```python
from build123d import *

# Parameters (mm, degrees)
F0_W     = 50.8
F0_H     = 38.1
F1_DEPTH = 25.4
F2_R     = 6.35
F3_DEPTH = 11.938
F4_R     = 8.89
F5_DEPTH = 6.35


with BuildPart() as f1:
    # F0 (on Front) → F1 (new body)
    with BuildSketch(Plane.XZ):
        with Locations((-25.4, -19.05)):
            Rectangle(F0_W, F0_H)
    extrude(amount=F1_DEPTH)

    # F2 (on Top) → F3 (join)
    with BuildSketch(Plane.XY):
        with Locations((-42.16706, -9.784626)):
            Circle(F2_R)
        with Locations((-20.268146, -10.25056)):
            Circle(F2_R)
    extrude(amount=F3_DEPTH)

    # F4 (on Front) → F5 (join)
    with BuildSketch(Plane.XZ):
        with Locations((-15.375839, -19.802213)):
            Circle(F4_R)
        with Locations((-37.274752, -19.802213)):
            Circle(F4_R)
    extrude(amount=-F5_DEPTH)


solid = f1.part
```
Part model, mm, in its own coordinate system. A direction names the side the tool comes from. Round coordinates to 2 decimals unless told otherwise and drop trailing zeros. Order: outer loops, then holes, each group sorted by start corner. A loop starts at its lowest first (then second) coordinate and runs counter-clockwise, first axis right, second up. Notation, with made-up numbers: M 55,88.5 L 75,88.5 A29 ccw 75,112.5 Z; hole C 67,66 d9. An arc over 180 degrees is marked long. Put each result on its own line as item: value. Start each with the question number.
1. Slice it at D-D on z = 3. List the corners of the cut face in (x, y), then the cut area to 3 significant figures.
2. Slice it at B-B on y = -6.5. List the corners of the cut face in (x, z), then the cut area to 3 significant figures.
3. Drop flat-ended pins along their axis: pin 1 (2 mm diameter, centred on x = -6.5, z = -8, fed in from +Y); pin 2 (10 mm diameter, centred on x = -6, y = -13, fed in from +Z). Give the stop position or say it passes through.
4. Slice it at C-C on y = 3.5. List the corners of the cut face in (x, z).
5. Slice it at A-A on x = -19.5. List the corners of the cut face in (y, z), then the cut area to 3 significant figures.
6. Tool access for faces 1 (the face through (-42, -10, 11.938)), 2 (the face through (-46.156, 3.131, -19.411)), 3 (the face through (-36.301, -12.217, 5.885)): list every direction of +Z, -Z, +X, -X, +Y, -Y with a clear straight run to the whole face (end or side of a thin tool).
7. Drill centre lines: probe 1 along Y at (x, z) = (-3, -27); probe 2 along Z at (x, y) = (-34, -16.5); probe 3 along X at (y, z) = (-14.5, 10). Where is each one in solid material? Low to high. Write a range as [from, to].
Findings:
1. outline: C -42.17,-9.78 d12.7; C -20.27,-10.25 d12.7
1. area: 253 mm2
2. outline: M -50.8,-38.1 L 0,-38.1 L 0,0 L -15.14,0 L -15.14,11.94 L -25.39,11.94 L -25.39,0 L -36.73,0 L -36.73,11.94 L -47.6,11.94 L -47.6,0 L -50.8,0 Z
2. area: 2,190 mm2
3. pin 1: y = 0
3. pin 2: z = 0
4. outline: C -37.27,-19.8 d17.78; C -15.38,-19.8 d17.78
5. outline: M -25.4,-38.1 L 0,-38.1 L 0,-27.68 L 6.35,-27.68 L 6.35,-11.93 L 0,-11.93 L 0,0 L -3.95,0 L -3.95,11.94 L -16.55,11.94 L -16.55,0 L -25.4,0 Z
5. area: 1,220 mm2
6. face 1: +Z, +X, -X, +Y, -Y
6. face 2: +Y
6. face 3: +Z
7. probe 1: [-25.4, 0]
7. probe 2: [-38.1, 0]
7. probe 3: [-46.42, -37.91], [-24.99, -15.55]
